Geometry check sheet. Reference: the model listing, model coordinates, mm. Coordinates: 2 decimals unless noted, no trailing zeros. Loops run counter-clockwise (first coordinate to the right, second up) from the corner with the lowest first, then second, coordinate; pieces in that order, holes last.
from build123d import *

# Parameters (mm, degrees)
SKETCH1_W           = 101.6
SKETCH1_H           = 95.25
BOSS_EXTRUDE1_DEPTH = 6.35
SKETCH2_W           = 12.7
SKETCH2_H           = 6.35
SKETCH2_R           = 1.651
SKETCH2_W_2         = 6.35
SKETCH2_H_2         = 12.7
BOSS_EXTRUDE2_DEPTH = 6.35
CUT_EXTRUDE1_DEPTH  = 80.746567925
LPATTERN1_COUNT     = 9
LPATTERN1_PITCH     = 9.525


with BuildPart() as part:
    # Sketch1 → Boss-Extrude1 (new body)
    with BuildSketch(Plane.XY):
        with Locations((0, -7.629593436)):
            Rectangle(SKETCH1_W, SKETCH1_H)
    extrude(amount=BOSS_EXTRUDE1_DEPTH)

    # Sketch2 → Boss-Extrude2 (add)
    # profile 1 of 6: a face of its own
    with BuildSketch(Plane.XY.offset(6.35)):
        with Locations((-25.4, 43.170406564)):
            Rectangle(SKETCH2_W, SKETCH2_H)
        with Locations((-25.4, 43.170406564)):
            Circle(SKETCH2_R, mode=Mode.SUBTRACT)
    # profile 2 of 6: a face of its own
    with BuildSketch(Plane.XY.offset(6.35)):
        with Locations((25.4, 43.170406564)):
            Rectangle(SKETCH2_W, SKETCH2_H)
        with Locations((25.4, 43.170406564)):
            Circle(SKETCH2_R, mode=Mode.SUBTRACT)
    # profile 3 of 6: a face of its own
    with BuildSketch(Plane.XY.offset(6.35)):
        with Locations((-53.975, 14.595406564)):
            Rectangle(SKETCH2_W_2, SKETCH2_H_2)
        with Locations((-53.975, 14.595406564)):
            Circle(SKETCH2_R, mode=Mode.SUBTRACT)
    # profile 4 of 6: a face of its own
    with BuildSketch(Plane.XY.offset(6.35)):
        with Locations((53.975, 14.595406564)):
            Rectangle(SKETCH2_W_2, SKETCH2_H_2)
        with Locations((53.975, 14.595406564)):
            Circle(SKETCH2_R, mode=Mode.SUBTRACT)
    # profile 5 of 6: a face of its own
    with BuildSketch(Plane.XY.offset(6.35)):
        with Locations((-53.975, -23.504593436)):
            Rectangle(SKETCH2_W_2, SKETCH2_H_2)
        with Locations((-53.975, -23.504593436)):
            Circle(SKETCH2_R, mode=Mode.SUBTRACT)
    # profile 6 of 6: a face of its own
    with BuildSketch(Plane.XY.offset(6.35)):
        with Locations((53.975, -23.504593436)):
            Rectangle(SKETCH2_W_2, SKETCH2_H_2)
        with Locations((53.975, -23.504593436)):
            Circle(SKETCH2_R, mode=Mode.SUBTRACT)
    extrude(amount=-BOSS_EXTRUDE2_DEPTH)

    # Sketch3 → Cut-Extrude1 (cut, through all)
    with BuildSketch(Plane.XY.offset(6.35)):
        with BuildLine():
            Line((-38.1, 33.645406564), (38.1, 33.645406564))
            ThreePointArc((38.1, 33.645406564), (41.275, 30.470406564), (38.1, 27.295406564))
            Line((38.1, 27.295406564), (-38.1, 27.295406564))
            ThreePointArc((-38.1, 27.295406564), (-41.275, 30.470406564), (-38.1, 33.645406564))
        make_face()
    cut_extrude1 = extrude(amount=-CUT_EXTRUDE1_DEPTH, mode=Mode.SUBTRACT)

    # LPattern1: Cut-Extrude1 ×9
    with Locations(*[(0, -i * LPATTERN1_PITCH, 0) for i in range(1, LPATTERN1_COUNT)]):
        add(cut_extrude1, mode=Mode.SUBTRACT)


solid = part.part
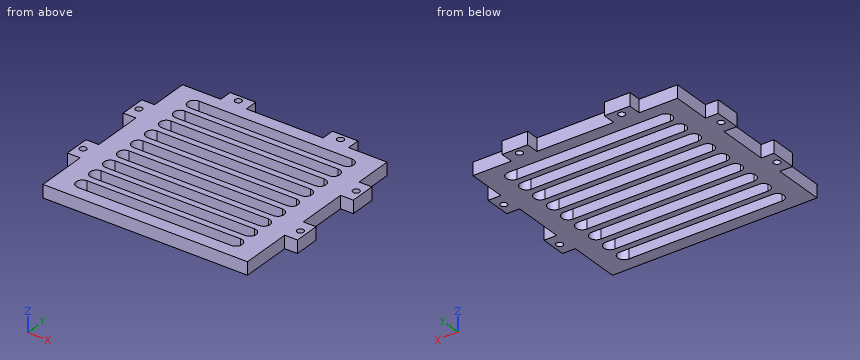
1) Section check D-D on y = -37. Record the cut outline in (x, z).
Data:
outline: (-50.8, 0) - (-41.17, 0) - (-41.17, 6.35) - (-50.8, 6.35) - close; (41.17, 0) - (50.8, 0) - (50.8, 6.35) - (41.17, 6.35) - close
2) Material ranges on probe 1 along Y at (x, z) = (-51, 3.75); probe 2 along X at (y, z) = (11, 4); probe 3 along X at (y, z) = (-36, 1.75), recorded low to high.
Data:
probe 1: y = -29.85 to -17.15, 8.25 to 20.95
probe 2: x = -57.15 to -41.25, 41.25 to 57.15
probe 3: x = -50.8 to -41.27, 41.27 to 50.8
3) Section check B-B on x = -25.4. Count the separate pieces of the cut face and the enclosed holes in it, and give its area (3 significant figures).
Data:
separate pieces: 11
enclosed holes: 0
area: 261 mm2
4) Depth check by flat-ended pin: pin 1 (3 mm diameter, centred on x = -15, z = 2, fed in from +Y). Enter the tip coordinate at first touch or a pass-through.
Data:
pin 1: stops at y = 40
5) Section check A-A on y = 1. Record the cut outline in (x, z), and give its area (3 significant figures).
Data:
outline: (-50.8, 0) - (-41.15, 0) - (-41.15, 6.35) - (-50.8, 6.35) - close; (41.15, 0) - (50.8, 0) - (50.8, 6.35) - (41.15, 6.35) - close
area: 123 mm2
